The listing builds one solid part. Answer for the finished solid, in the listing's coordinates (mm). Face numbers are marked on the shaded views. A direction names the side the tool comes from. Round coordinates to 2 decimals unless told otherwise and drop trailing zeros. Order: outer loops, then holes, each group sorted by start corner. A loop starts at its lowest first (then second) coordinate and runs counter-clockwise, first axis right, second up. Notation, with made-up numbers: (70.25, 44.25) -> (74.25, 44.25) arc R10 ccw to (74.25, 52.25) -> close; hole circle Ø6 at (66.5, 25.5). An arc over 180 degrees is marked (long way). Return JSON: item names as keys, results as strings. Group by question number.
(1) The part is cut by section D-D (x = 10). Determine the outline of the cut face in (y, z), plus the area to 3 significant figures.
(2) Each of these flat-tipped pins is pushed along its axis until it touches: pin 1 (2 mm diameter, centred on x = 9, y = -0.5, fed in from +Z); pin 2 (0.6 mm diameter, centred on y = -2, z = -1.5, fed in from -X); pin 3 (3 mm diameter, centred on x = 9.5, z = 1, fed in from +Y); pin 4 (3 mm diameter, centred on x = 5, z = -2.5, fed in from +Y). Where does it stop, or does it pass through?
(3) Which of the six approach directions +Z, -Z, +X, -X, +Y, -Y give full straight-line access (tool end or side, diameter ignored) to the marked faces 1 and 2?
(4) The part is cut by section B-B (x = 5). Determine the outline of the cut face in (y, z), plus the area to 3 significant figures.
(5) The part is cut by section A-A (z = 0). Determine the outline of the cut face in (x, y), plus the area to 4 significant figures.
(6) Consider line 1 (X direction, y = -2, z = 2); line 2 (Y direction, x = 3.35, z = 0); line 3 (X direction, y = 0.5, z = -0.5). Determine where each line is inside the solid, lowest interval first. Write a range as [from, to].
(7) The part is cut by section C-C (y = -1.25). Determine the outline of the cut face in (x, z), plus the area to 3 significant figures.
(8) Determine the mould class of the marked faces 3, 4 and 5 for opening direction X: +X half, -X half, draft (parallel to the pull), parting line (faces both ways), or undercut.
from build123d import *

# Parameters (mm, degrees)
CUT_EXTRUDE6_DEPTH = 4
SKETCH5_R          = 2.2
CUT_EXTRUDE7_DEPTH = 5.5


with BuildPart() as part:
    # Sketch3 → Revolve5 (revolve)
    with BuildSketch(Plane.XY, mode=Mode.PRIVATE) as revolve5_sk:
        Polygon((0, 0), (0, 3.25), (1.5, 3.25), (1.5, 2.4), (10.5, 2.4), (10.5, 2.9), (11, 2.9), (11, 0), align=None)
    revolve(revolve5_sk.sketch.rotate(Axis((11, 0, 0), (-1, 0, 0)), 90), axis=Axis((11, 0, 0), (-1, 0, 0)))

    # Sketch4 → Cut-Extrude6 (cut)
    with BuildSketch(Plane(origin=(11, 0, 0), x_dir=(0, 0, -1), z_dir=(1, 0, 0))):
        with BuildLine():
            ThreePointArc((-0.5, -2.856571371), (-0.250941252, -2.889122443), (-3e-09, -2.9))
            ThreePointArc((-3e-09, -2.9), (0.25094125, -2.889122443), (0.5, -2.856571371))
            Line((0.5, -2.856571371), (0.5, -2.142428529))
            ThreePointArc((0.5, -2.142428529), (0, -2.2), (-0.5, -2.142428529))
            Line((-0.5, -2.142428529), (-0.5, -2.856571371))
        make_face()
        with BuildLine():
            Line((-0.5, 2.856571371), (-0.5, 2.142428529))
            ThreePointArc((-0.5, 2.142428529), (0, 2.2), (0.5, 2.142428529))
            Line((0.5, 2.142428529), (0.5, 2.856571371))
            ThreePointArc((0.5, 2.856571371), (0.250941244, 2.889122443), (-1.4e-08, 2.9))
            ThreePointArc((-1.4e-08, 2.9), (-0.250941258, 2.889122442), (-0.5, 2.856571371))
        make_face()
        with BuildLine():
            Line((-0.5, 2.142428529), (-0.5, -2.142428529))
            ThreePointArc((-0.5, -2.142428529), (0, -2.2), (0.5, -2.142428529))
            Line((0.5, -2.142428529), (0.5, 2.142428529))
            ThreePointArc((0.5, 2.142428529), (0, 2.2), (-0.5, 2.142428529))
        make_face()
        with BuildLine():
            ThreePointArc((-0.5, 2.142428529), (-2.2, 0), (-0.5, -2.142428529))
            Line((-0.5, -2.142428529), (-0.5, 2.142428529))
        make_face()
        with BuildLine():
            Line((0.5, 2.142428529), (0.5, -2.142428529))
            ThreePointArc((0.5, -2.142428529), (1.723368794, -1.367479433), (2.2, 0))
            ThreePointArc((2.2, 0), (1.723368794, 1.367479433), (0.5, 2.142428529))
        make_face()
        with BuildLine():
            Line((2.4, 1.62788206), (2.4, -1.62788206))
            ThreePointArc((2.4, -1.62788206), (2.772183255, -0.851469318), (2.9, 0))
            ThreePointArc((2.9, 0), (2.772183255, 0.851469318), (2.4, 1.62788206))
        make_face()
        with BuildLine():
            ThreePointArc((-2.9, -6e-09), (-2.772183254, -0.851469321), (-2.4, -1.62788206))
            Line((-2.4, -1.62788206), (-2.4, 1.62788206))
            ThreePointArc((-2.4, 1.62788206), (-2.772183256, 0.851469315), (-2.9, -6e-09))
        make_face()
    extrude(amount=-CUT_EXTRUDE6_DEPTH, mode=Mode.SUBTRACT)

    # Sketch5 → Cut-Extrude7 (cut)
    with BuildSketch(Plane(origin=(7, 0, 0), x_dir=(0, 0, -1), z_dir=(1, 0, 0))):
        Circle(SKETCH5_R)
    extrude(amount=-CUT_EXTRUDE7_DEPTH, mode=Mode.SUBTRACT)


solid = part.part
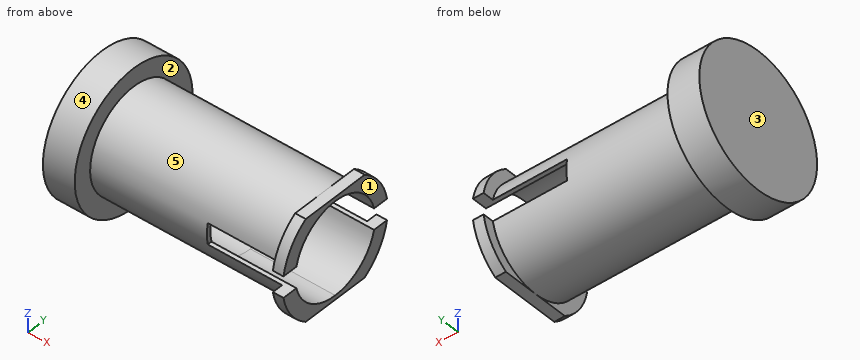
Answer below:
{
 "1": {"outline": "(-2.35, -0.5) arc R2.4 ccw to (2.35, -0.5) -> (2.14, -0.5) arc R2.2 cw to (-2.14, -0.5) -> close; (-2.35, 0.5) -> (-2.14, 0.5) arc R2.2 cw to (2.14, 0.5) -> (2.35, 0.5) arc R2.4 ccw to start", "area": "2.49 mm²"},
 "2": {"pin 1": "stops at z = 2.4", "pin 2": "stops at x = 0", "pin 3": "stops at y = 2.86", "pin 4": "stops at y = 2.18"},
 "3": {"face 1": "+Z, -Z, +X, +Y, -Y", "face 2": "none"},
 "4": {"outline": "circle Ø4.8 at (0, 0); hole circle Ø4.4 at (0, 0)", "area": "2.89 mm²"},
 "5": {"outline": "(0, -3.25) -> (1.5, -3.25) -> (1.5, -2.4) -> (7, -2.4) -> (7, -2.2) -> (1.5, -2.2) -> (1.5, 2.2) -> (7, 2.2) -> (7, 2.4) -> (1.5, 2.4) -> (1.5, 3.25) -> (0, 3.25) -> close", "area": "11.95 mm²"},
 "6": {"line 1": "x = [0, 1.5], [10.5, 11]", "line 2": "y = [-2.4, -2.2], [2.2, 2.4]", "line 3": "x = [0, 1.5]"},
 "7": {"outline": "(0, -3) -> (1.5, -3) -> (1.5, -2.05) -> (10.5, -2.05) -> (10.5, -2.4) -> (11, -2.4) -> (11, -1.81) -> (1.5, -1.81) -> (1.5, 1.81) -> (11, 1.81) -> (11, 2.4) -> (10.5, 2.4) -> (10.5, 2.05) -> (1.5, 2.05) -> (1.5, 3) -> (0, 3) -> close", "area": "13.9 mm²"},
 "8": {"face 3": "-X half", "face 4": "draft", "face 5": "undercut"}
}
